Input: part model. Units: mm. Frame: model coordinates. Give positions to 0.01 mm unless a question says otherwise; leave off trailing zeros. Loops run counter-clockwise (first coordinate to the right, second up) from the corner with the lowest first, then second, coordinate; pieces in that order, holes last. Notation, with made-up numbers: (73.25, -20.5) -> (116.25, -20.5) arc R20 cw to (116.25, -1.5) -> close; hole circle Ø3 at (76, -2). An arc over 180 degrees is marked (long way). Answer in a Markdown table with one row per item. Add a question column.
```python
from build123d import *

# Parameters (mm, degrees)
EXTRUDE_1_DEPTH         = 5
FILLET_1_R              = 3
SKETCH_2_R              = 2
SKETCH_2_R_2            = 4.5
CUT_EXTRUDE_1_DEPTH     = 106.594744187
HOLE_WIZARD_M10_5_D     = 10
HOLE_WIZARD_M10_5_DEPTH = 24.5


with BuildPart() as part:
    # 草图1 → 凸台-拉伸1 (new body)
    with BuildSketch(Plane.XY):
        Polygon((-35, 0), (0, 0), (0, 50), (-5.5, 99.5), (-29.5, 99.5), (-35, 50), align=None)
    extrude(amount=EXTRUDE_1_DEPTH)

    # 圆角1
    fillet_1_edges = [part.edges().sort_by_distance(p)[0] for p in [
        (-35, 50, 2.5),
        (-29.5, 99.5, 2.5),
        (-5.5, 99.5, 2.5),
        (0, 50, 2.5),
        (0, 0, 2.5),
        (-35, 0, 2.5),
    ]]
    fillet(fillet_1_edges, radius=FILLET_1_R)

    # 草图2 → 切除-拉伸1 (cut, through all)
    with BuildSketch(Plane.XY.offset(5)):
        with Locations((-29.5, 6)):
            Circle(SKETCH_2_R)
        with Locations((-17.5, 6)):
            Circle(SKETCH_2_R)
        with Locations((-5.5, 6)):
            Circle(SKETCH_2_R)
        with Locations((-17.5, 89.5)):
            Circle(SKETCH_2_R_2)
        with Locations((-17.5, 69.5)):
            Circle(SKETCH_2_R_2)
    extrude(amount=-CUT_EXTRUDE_1_DEPTH, mode=Mode.SUBTRACT)

    # M10 螺纹孔5
    with Locations(Plane.XY.offset(5)):
        with Locations((-17.5, 69.5), (-17.5, 89.5)):
            Hole(HOLE_WIZARD_M10_5_D / 2, depth=HOLE_WIZARD_M10_5_DEPTH)


solid = part.part
```
1) Pull-direction query (Y, two-part tool) for faces 1 (the face through (-6.974, 7.352, 2.535)), 2 (the face through (-6.162, 98.715, 2.535)), 3 (the face through (-0.9, 0.86, 2.54)); classes: +Y half, -Y half, draft (parallel to the pull), parting line (faces both ways), or undercut.
2) Pin query (flat end, axial travel): pin 1 (5 mm diameter, centred on x = -12.5, y = 30.5, fed in from -Z); pin 2 (3.5 mm diameter, centred on x = -5.5, y = 6, fed in from -Z). Return the tip coordinate at first contact, or that it passes through.
3) Section D-D on y = 89.5. Output: boundary loops of the cut face in (x, z).
4) Material intervals for line 1 along Y through (x, z) = (-17.5, 2.25); line 2 along Y through (x, z) = (-13.5, 0.4); line 3 along Y through (x, z) = (-18.5, 3.55), sorted ascending.
5) Section C-C on z = 3. Output: boundary loops of the cut face in (x, y).
6) Section B-B on y = 6. Output: boundary loops of the cut face in (x, z), and give its area (3 significant figures).
7) Section A-A on x = -17.5. Output: boundary loops of the cut face in (y, z), and give its area (4 significant figures).
Working result:
| question | item | result |
|---|---|---|
| 1 | face 1 | undercut |
| 1 | face 2 | +Y half |
| 1 | face 3 | -Y half |
| 2 | pin 1 | stops at z = 0 |
| 2 | pin 2 | passes through |
| 3 | outline | (-30.61, 0) -> (-22.5, 0) -> (-22.5, 5) -> (-30.61, 5) -> close; (-12.5, 0) -> (-4.39, 0) -> (-4.39, 5) -> (-12.5, 5) -> close |
| 4 | line 1 | y = 0 to 4, 8 to 64.5, 74.5 to 84.5, 94.5 to 99.5 |
| 4 | line 2 | y = 0 to 66.5, 72.5 to 86.5, 92.5 to 99.5 |
| 4 | line 3 | y = 0 to 4.27, 7.73 to 64.6, 74.4 to 84.6, 94.4 to 99.5 |
| 5 | outline | (-35, 3) arc R3 ccw to (-32, 0) -> (-3, 0) arc R3 ccw to (0, 3) -> (0, 49.83) arc R3 ccw to (-0.02, 50.17) -> (-5.2, 96.83) arc R3 ccw to (-8.19, 99.5) -> (-26.81, 99.5) arc R3 ccw to (-29.8, 96.83) -> (-34.98, 50.17) arc R3 ccw to (-35, 49.83) -> close; hole circle Ø4 at (-29.5, 6); hole circle Ø10 at (-17.5, 69.5); hole circle Ø10 at (-17.5, 89.5); hole circle Ø4 at (-17.5, 6); hole circle Ø4 at (-5.5, 6) |
| 6 | outline | (-35, 0) -> (-31.5, 0) -> (-31.5, 5) -> (-35, 5) -> close; (-27.5, 0) -> (-19.5, 0) -> (-19.5, 5) -> (-27.5, 5) -> close; (-15.5, 0) -> (-7.5, 0) -> (-7.5, 5) -> (-15.5, 5) -> close; (-3.5, 0) -> (0, 0) -> (0, 5) -> (-3.5, 5) -> close |
| 6 | area | 115 mm2 |
| 7 | outline | (0, 0) -> (4, 0) -> (4, 5) -> (0, 5) -> close; (8, 0) -> (64.5, 0) -> (64.5, 5) -> (8, 5) -> close; (74.5, 0) -> (84.5, 0) -> (84.5, 5) -> (74.5, 5) -> close; (94.5, 0) -> (99.5, 0) -> (99.5, 5) -> (94.5, 5) -> close |
| 7 | area | 377.5 mm2 |
